Autodesk Inventor part; units mm, degrees
ref_plane "YZ Plane" through (0, 0, 0) normal (1, 0, 0) x (0, 1, 0)
ref_plane "XZ Plane" through (0, 0, 0) normal (0, 1, 0) x (-1, 0, 0)
ref_plane "XY Plane" through (0, 0, 0) normal (0, 0, 1) x (1, 0, 0)
sketch "Sketch1" plane through (0, 0, 0) normal (0, 1, 0) x (-1, 0, 0)
  line L0 (0, 0) -> (70, 0)
  line L1 (70, 0) -> (70, -110)
  line L2 (70, -110) -> (0, -110)
  line L3 (0, -110) -> (0, 0)
  line L4 (2.5, -2.5) -> (67.5, -2.5)
  line L5 (67.5, -2.5) -> (67.5, -107.5)
  line L6 (67.5, -107.5) -> (2.5, -107.5)
  line L7 (2.5, -107.5) -> (2.5, -2.5)
  line L8 (2.5, -2.5) -> (67.5, -107.5) construction
  line L9 (67.5, -2.5) -> (2.5, -107.5) construction
  point P0 (35, -55)
  dimension "d0" = 70
  dimension "d1" = 110
  dimension "d2" = 65
  dimension "d3" = 105
extrude "Extrusion1" add sketch "Sketch1" along normal blind 30
sketch "Sketch2" plane through (0, 0, 0) normal (0, -1, 0) x (1, 0, 0)
  line L0 (0, -110) -> (-70, -110)
  line L1 (0, 0) -> (-70, 0)
  line L2 (-70, 0) -> (-70, -110)
  line L3 (-70, -110) -> (0, -110)
  line L4 (0, -110) -> (0, 0)
extrude "Extrusion2" add sketch "Sketch2" against normal blind 3
sketch "Sketch3" plane through (0, 0, 0) normal (0, -1, 0) x (1, 0, 0)
  line L0 (-2.5, -107.5) -> (-2.5, -2.5)
  line L1 (-2.5, -107.5) -> (-46.5, -107.5)
  line L2 (-46.5, -107.5) -> (-46.5, -29.5)
  line L3 (-46.5, -29.5) -> (-2.5, -29.5)
  line L4 (-2.5, -29.5) -> (-2.5, -107.5)
  line L5 (-45.25, -106.5) -> (-3.75, -106.5)
  line L6 (-3.75, -106.5) -> (-3.75, -30.5)
  line L7 (-3.75, -30.5) -> (-45.25, -30.5)
  line L8 (-45.25, -30.5) -> (-45.25, -106.5)
  line L9 (-45.25, -106.5) -> (-3.75, -30.5) construction
  line L10 (-3.75, -106.5) -> (-45.25, -30.5) construction
  point P0 (0, 0)
  point P1 (-24.5, -68.5)
  dimension "d8" = 44
  dimension "d9" = 78
  dimension "d10" = 41.5
  dimension "d11" = 76
extrude "Extrusion3" add sketch "Sketch3" against normal blind 25
extrude "Extrusion4" cut sketch "Sketch3" against normal blind 25 contours L8 L7 L6 L5
sketch "Sketch4" plane through (0, 25, 0) normal (0, 1, 0) x (1, 0, 0)
  line L0 (-46.5, 107.5) -> (-46.5, 29.5)
  line L1 (-2.5, 107.5) -> (-2.5, 29.5)
  line L2 (-46.5, 29.5) -> (-2.5, 29.5)
  line L3 (-2.5, 29.5) -> (-2.5, 107.5)
  line L4 (-2.5, 107.5) -> (-46.5, 107.5)
  line L5 (-46.5, 107.5) -> (-46.5, 29.5)
  point P0 (0, 0)
  point P1 (-2.5, 29.5)
extrude "Extrusion5" add sketch "Sketch4" against normal blind 2
fillet "Fillet1" radius 2 3 edges at (-46.5, 25, -68.5) (-46.5, 14, -29.5) (-24.5, 25, -29.5)
sketch "Sketch5" plane through (0, 23, 0) normal (0, -1, 0) x (1, 0, 0)
  line L0 (-45.25, -30.5) -> (-3.75, -30.5) construction
  line L1 (-3.75, -30.5) -> (-3.75, -106.5) construction
  line L2 (-45.25, -30.5) -> (-3.75, -106.5) construction
  line L3 (-3.75, -106.5) -> (-45.25, -106.5) construction
  line L4 (0, 0) -> (0, -110) construction
  line L5 (-45.25, -106.5) -> (-3.75, -30.5) construction
  line L6 (-24.5, -68.5) -> (-24.5, -106.5) construction
  line L7 (-3.75, -106.5) -> (-45.25, -106.5) construction
  line L8 (-24.5, -68.5) -> (-24.5, -30.5) construction
  line L9 (-45.25, -106.5) -> (-24.5, -30.5) construction
  line L10 (-45.25, -30.5) -> (-24.5, -106.5) construction
  line L11 (-24.5, -106.5) -> (-3.75, -30.5) construction
  line L12 (-24.5, -30.5) -> (-3.75, -106.5) construction
  line L13 (-31.875, -68.5) -> (-37.875, -68.5) construction
  line L14 (-31.875, -67.75) -> (-37.875, -67.75)
  line L15 (-37.875, -69.25) -> (-31.875, -69.25)
  arc A0 (-31.875, -69.25) -> (-31.875, -67.75) centre (-31.875, -68.5) ccw
  arc A1 (-37.875, -67.75) -> (-37.875, -69.25) centre (-37.875, -68.5) ccw
  line L16 (-11.125, -68.5) -> (-17.125, -68.5) construction
  line L17 (-11.125, -67.75) -> (-17.125, -67.75)
  line L18 (-17.125, -69.25) -> (-11.125, -69.25)
  arc A2 (-11.125, -69.25) -> (-11.125, -67.75) centre (-11.125, -68.5) ccw
  arc A3 (-17.125, -67.75) -> (-17.125, -69.25) centre (-17.125, -68.5) ccw
  point P0 (-34.875, -68.5)
  point P1 (-14.125, -68.5)
  dimension "d19" = 3
  dimension "d20" = 1.5
  dimension "d21" = 3
  dimension "d22" = 1.5
extrude "Extrusion6" cut sketch "Sketch5" against normal blind 2
sketch "Sketch6" plane through (-44.5, 23, -29.5) normal (0, 0, 1) x (1, 0, 0)
  line L0 (44.5, 7) -> (44.5, -23)
  line L1 (44.5, -23) -> (-25.5, -23)
  line L2 (-25.5, -23) -> (-25.5, 7)
  line L3 (-25.5, 7) -> (-23, 7)
  line L4 (-23, 7) -> (-23, -20)
  line L5 (-23, -20) -> (0, -20)
  line L6 (0, -20) -> (0, 0)
  line L7 (0, 0) -> (42, 0)
  line L8 (42, -20) -> (42, 0)
  line L9 (0, -20) -> (42, -20)
  line L10 (42, 7) -> (44.5, 7)
  line L11 (42, 0) -> (42, 7)
  line L12 (42, 0) -> (0, -20) construction
  line L13 (42, -20) -> (0, 0) construction
  line L14 (18, -10) -> (24, -10) construction
  line L15 (18, -11) -> (24, -11)
  line L16 (24, -9) -> (18, -9)
  arc A0 (18, -9) -> (18, -11) centre (18, -10) ccw
  arc A1 (24, -11) -> (24, -9) centre (24, -10) ccw
  point P0 (21, -10)
  dimension "d25" = 3
  dimension "d26" = 2
extrude "Extrusion7" cut sketch "Sketch6" against normal blind 2 contours A0 L16 A1 L15
sketch "Sketch7" plane through (0, 30, 0) normal (0, 1, 0) x (1, 0, 0)
  line L0 (-67.5, 107.5) -> (-46.5, 107.5)
  circle A0 centre (-67.5, 107.5) radius 2.5
  line L1 (0, 110) -> (-70, 110)
  line L2 (-2.5, 2.5) -> (-67.5, 2.5)
  circle A1 centre (-2.5, 2.5) radius 2.5
  line L3 (-70, 0) -> (0, 0)
  circle A2 centre (-67.5, 2.5) radius 2.5
extrude "Extrusion8" add sketch "Sketch7" against normal blind 30 contours A0 | A1 | A2
fillet "Fillet2" radius 2 3 edges at (0, 15, 0) (-70, 15, 0) (-70, 15, -110)
sketch "Sketch8" plane through (0, 30, 0) normal (0, 1, 0) x (1, 0, 0)
  arc A0 (-65, 2.5) -> (-67.5, 5) centre (-67.5, 2.5) ccw
  arc A1 (-2.5, 5) -> (-5, 2.5) centre (-2.5, 2.5) ccw
  arc A2 (-67.5, 105) -> (-65, 107.5) centre (-67.5, 107.5) ccw
  point P0 (0, 0)
hole "Hole1" at (-67.5, 30, -2.5) at (-2.5, 30, -2.5) at (-67.5, 30, -107.5) direction (0, -1, 0) diameter 3 depth 40 tip angle 118
fillet "Fillet3" radius 2 1 edges at (0, 15, -110)
sketch "Sketch9" plane through (-45.25, 0, -106.5) normal (0, 0, 1) x (1, 0, 0)
  line L0 (-24.75, 30) -> (-23.368, 30)
  line L1 (-23.368, 30) -> (-23.368, 0)
  line L2 (-23.368, 0) -> (-24.75, 0)
  line L3 (-24.75, 0) -> (-24.75, 30)
  line L4 (41.5, 23) -> (0, 23)
  line L5 (0, 23) -> (0, 0)
  line L6 (0, 0) -> (-21.132, 0)
  line L7 (-21.132, 0) -> (-21.132, 30)
  line L8 (-21.132, 30) -> (-19.9587, 30)
  line L9 (-19.9587, 30) -> (-19.9587, 3)
  line L10 (-19.9587, 3) -> (-1.25, 3)
  line L11 (-1.25, 3) -> (-1.25, 23)
  arc A0 (0.75, 25) -> (-1.25, 23) centre (0.75, 23) ccw
  line L12 (0.75, 25) -> (42.75, 25)
  line L13 (42.75, 25) -> (42.75, 30)
  line L14 (42.75, 30) -> (45.25, 30)
  line L15 (45.25, 30) -> (45.25, 0)
  line L16 (45.25, 0) -> (41.5, 0)
  line L17 (41.5, 0) -> (0, 0)
  line L18 (41.5, 0) -> (41.5, 23)
  line L19 (0, 3) -> (2, 3) construction
  line L20 (-19.75, 3) -> (-1.25, 3) construction
  line L21 (2, 3) -> (4, 3)
  line L22 (4, 3) -> (4, 1)
  line L23 (4, 1) -> (2, 1)
  line L24 (2, 1) -> (2, 3)
  line L25 (41.5, 3) -> (39.5, 3) construction
  line L26 (39.5, 3) -> (37.5, 3)
  line L27 (37.5, 3) -> (37.5, 1)
  line L28 (37.5, 1) -> (39.5, 1)
  line L29 (39.5, 1) -> (39.5, 3)
  dimension "d40" = 2
  dimension "d41" = 2
  dimension "d42" = 2
  dimension "d43" = 2
  dimension "d44" = 2
  dimension "d45" = 2
extrude "Extrusion9" cut sketch "Sketch9" against normal blind 2 contours L21 L22 L23 L24 | L29 L28 L27 L26
sketch "Sketch10" plane through (0, 0, 0) normal (0, -1, 0) x (1, 0, 0)
  line L0 (-45.25, -30.5) -> (-3.75, -30.5)
  circle A0 centre (-24.5, -30.5) radius 7.5
  point P0 (0, 0)
  point P1 (-17, -30.5)
  point P2 (-32, -30.5)
  dimension "d48" = 15
extrude "Extrusion10" cut sketch "Sketch10" against normal blind 1.5 contours A0 L0 picked at (-23.8998, -27.0007)
sketch "Sketch12" plane through (0, 1.5, 0) normal (0, -1, 0) x (1, 0, 0)
  arc A0 (-17, -30.5) -> (-32, -30.5) centre (-24.5, -30.5) ccw construction
  line L0 (-24.5, -30.5) -> (-24.5, -26.75) construction
  line L1 (-24.5, -30.5) -> (-20.75, -30.5) construction
  point P0 (0, 0)
  dimension "d58" = 3.75
  dimension "d59" = 90
hole "Hole3" at (-24.5, 1.5, -26.75) direction (0, 1, 0) diameter 1 depth 1 tip angle 118
sketch "Sketch14" plane through (-70, 0, -108) normal (-1, 0, 0) x (0, 0, 1)
  line L0 (0, 0) -> (0, 30) construction
  line L1 (108, 0) -> (106, 0) construction
  line L2 (106, 0) -> (106, 30) construction
  line L3 (108, 30) -> (108, 0) construction
  line L4 (53, 15) -> (106, 15) construction
  line L5 (106, 0) -> (106, 30) construction
  line L6 (53, 15) -> (0, 15) construction
  line L7 (0, 15) -> (17.6, 15) construction
  point P0 (35.2, 15)
  point P1 (52.8, 15)
  point P2 (70.4, 15)
  point P3 (88, 15)
  dimension "d71" = 17.6
  dimension "d74" = 17.6
  dimension "d79" = 18
hole "Hole4" at (-70, 15, -90.4) at (-70, 15, -72.8) at (-70, 15, -55.2) at (-70, 15, -37.6) at (-70, 15, -20) direction (1, 0, 0) diameter 5.5 depth 3
sketch "Sketch16" plane through (-68, 0, 0) normal (0, 0, 1) x (1, 0, 0)
  line L0 (0, 0) -> (66, 0) construction
  line L1 (66, 0) -> (62, 0) construction
  line L2 (66, 0) -> (70, 0) construction
  line L3 (62, 0) -> (62, 30) construction
  line L4 (0, 30) -> (66, 30) construction
  line L5 (62, 23.7699) -> (50, 23.7699)
  line L6 (50, 23.7699) -> (50, 4.7699)
  line L7 (50, 4.7699) -> (62, 4.7699)
  line L8 (62, 4.7699) -> (62, 23.7699)
  point P0 (68, 0)
  dimension "d88" = 4
  dimension "d89" = 180
  dimension "d90" = 12
  dimension "d91" = 19
extrude "Extrusion11" cut sketch "Sketch16" against normal blind 3
properties part number "inferior model2"
Read the model definition and answer for the solid it produces. Units are mm, in the model's axes. A direction names the side the tool comes from. Coordinates: 2 decimals unless noted, no trailing zeros. Write each loop counter-clockwise with the first axis right and the second up, starting at its lowest first coordinate (ties: lowest second). Pieces come first, ordered by that corner, then holes. Notation, with made-up numbers: (68, -9) - (122, -9) arc R20 ccw to (122, 13) - close; hole circle Ø3 at (62.5, 15.5). An arc over 180 degrees is marked (long way). Answer as a JSON object with one key per item and string values. Group by question number.
1. A cutting plane is placed at C-C (x = -58.5). Determine the outline of the cut face in (y, z), plus the area to 3 significant figures.
2. Each of these flat-tipped pins is pushed along its axis until it touches: P1, Ø1.8, axis at x = -67.5, z = -2.5, coming from the -Y side; P2, Ø3.5, axis at y = 15, z = -20, coming from the -X side; P3, Ø2, axis at x = -24.5, z = -45.5, coming from the +Y side; P4, Ø1.5, axis at x = -14, y = 7, coming from the +Z side. Where does it stop, or does it pass through?
3. A cutting plane is placed at A-A (z = -20). Determine the outline of the cut face in (x, y).
4. The mould has two halves that part along Y. Classify faces 1 (the flat face through (-24, 25, -69)), 2 (the flat face through (-6, 14, -1)), 3 (the cylindrical face through (-68.732, 14.879, -22.747)), 4 (the flat face through (-24, 11, -30.5)): +Y half, -Y half, draft (parallel to the pull), parting line (faces both ways), or undercut.
5. Consider L1, parallel to X at y = 20.25, z = -75.5; L2, parallel to Z at x = -23, y = 5; L3, parallel to X at y = 9.75, z = -20.5. Determine where each line is inside the solid, lowest interval first. Write a range as [from, to].
6. A cutting plane is placed at D-D (z = -66). Determine the outline of the cut face in (x, y).
7. A cutting plane is placed at B-B (y = 26.25). Determine the outline of the cut face in (x, z), plus the area to 3 significant figures.
8. Which of the six approach directions +Z, -Z, +X, -X, +Y, -Y give full straight-line access (tool end or side, diameter ignored) to faces 5 (the flat face through (-12, 23.77, -1)), 6 (the flat face through (-2.5, 25.3, -34.2)), 7 (the cylindrical face through (-68.732, 13.141, -39.627)), 8 (the cylindrical face through (-24.34, 0.74, -23))?
Worked out:
{
 "1": {"outline": "(0, -110) - (30, -110) - (30, -107.5) - (3, -107.5) - (3, -2.5) - (30, -2.5) - (30, 0) - (0, 0) - close", "area": "465 mm²"},
 "2": {"P1": "passes through", "P2": "stops at x = -2.5", "P3": "stops at y = 25", "P4": "stops at z = -29.5"},
 "3": {"outline": "(-70, 0) - (0, 0) - (0, 30) - (-2.5, 30) - (-2.5, 3) - (-67.5, 3) - (-67.5, 12.25) - (-70, 12.25) - close; (-70, 17.75) - (-67.5, 17.75) - (-67.5, 30) - (-70, 30) - close"},
 "4": {"face 1": "+Y half", "face 2": "undercut", "face 3": "undercut", "face 4": "draft"},
 "5": {"L1": "x = [-70, -67.5], [-46.5, -45.25], [-3.75, 0]", "L2": "z = [-110, -106.5], [-30.5, -29.5], [-2.5, 0]", "L3": "x = [-70, -67.5], [-2.5, 0]"},
 "6": {"outline": "(-70, 0) - (-45.25, 0) - (-45.25, 23) - (-3.75, 23) - (-3.75, 0) - (0, 0) - (0, 30) - (-2.5, 30) - (-2.5, 25) - (-44.5, 25) arc R2 ccw to (-46.5, 23) - (-46.5, 3) - (-67.5, 3) - (-67.5, 30) - (-70, 30) - close"},
 "7": {"outline": "(-70, -108) arc R2 ccw to (-68, -110) - (-2, -110) arc R2 ccw to (0, -108) - (0, -2) arc R2 ccw to (-2, 0) - (-68, 0) arc R2 ccw to (-70, -2) - close; hole circle Ø3 at (-67.5, -107.5); hole circle Ø3 at (-67.5, -2.5); hole (-67.5, -105) arc R2.5 cw to (-65, -107.5) - (-2.5, -107.5) - (-2.5, -5) arc R2.5 cw to (-5, -2.5) - (-65, -2.5) arc R2.5 cw to (-67.5, -5) - close; hole circle Ø3 at (-2.5, -2.5)", "area": "865 mm²"},
 "8": {"face 5": "+Z", "face 6": "+Y", "face 7": "-X", "face 8": "-Y"}
}
